from build123d import *

# Parameters (mm, degrees)
SKETCH008_R          = 10.15
SKETCH008_R_2        = 8.35
PAD006_DEPTH         = 55
SKETCH009_R          = 10.15
POCKET002_DEPTH      = 10.15
POCKET002_DEPTH_BACK = 10.15
SKETCH010_R          = 10.15
POCKET003_DEPTH      = 10.15
POCKET003_DEPTH_BACK = 10.15


with BuildPart() as part:
    # Sketch008 → Pad006 (new body)
    with BuildSketch(Plane.XY):
        Circle(SKETCH008_R)
        Circle(SKETCH008_R_2, mode=Mode.SUBTRACT)
    extrude(amount=PAD006_DEPTH)

    # Sketch009 → Pocket002 (cut, two sides)
    with BuildSketch(Plane.XZ) as pocket002_sk:
        Circle(SKETCH009_R)
    extrude(amount=-POCKET002_DEPTH, mode=Mode.SUBTRACT)
    extrude(pocket002_sk.sketch, amount=POCKET002_DEPTH_BACK, mode=Mode.SUBTRACT)

    # Sketch010 → Pocket003 (cut, two sides)
    with BuildSketch(Plane.YZ) as pocket003_sk:
        Circle(SKETCH010_R)
    extrude(amount=-POCKET003_DEPTH, mode=Mode.SUBTRACT)
    extrude(pocket003_sk.sketch, amount=POCKET003_DEPTH_BACK, mode=Mode.SUBTRACT)


solid = part.part
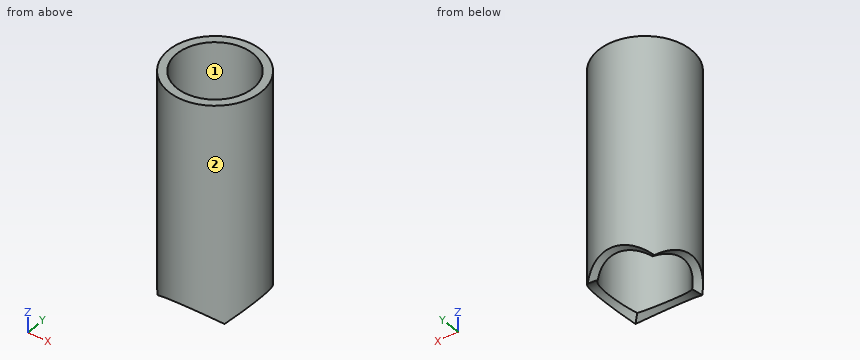
The listing builds one solid part. Answer for the finished solid, in the listing's coordinates (mm). Face numbers are marked on the shaded views. Round coordinates to 2 decimals unless told otherwise and drop trailing zeros. Order: outer loops, then holes, each group sorted by start corner. A loop starts at its lowest first (then second) coordinate and runs counter-clockwise, first axis right, second up. Notation, with made-up numbers: (-10, 12) - (-5, 12) arc R28 cw to (-5, 34) - close; hole circle Ø5 at (16, -29). An arc over 180 degrees is marked (long way). Write item = value, one per line. Start each with the question number.
1) Section B-B, the plane z = 43.5 is taken. Write down the section's boundary in (x, y), plus the area to 3 significant figures.
2) For a pull along X with two mould halves and no side action, classify the marked faces 1 and 2 as released by +X, released by -X, zero draft, split by the parting line, or undercut.
3) Given pin 1 (1 mm diameter, centred on y = -8, z = 29.5, fed in from -X); pin 2 (5 mm diameter, centred on x = -0.5, z = 40.5, fed in from -Y); pin 3 (1.5 mm diameter, centred on y = 3.5, z = 31, fed in from +X); pin 4 (1.5 mm diameter, centred on y = -2.5, z = 47, fed in from +X), each flat-ended and moving along its own axis, determine where each tip first touches the part or whether it passes through.
4) Straight lines are drawn through the part: L1, parallel to Y at x = 0, z = 18; L2, parallel to X at y = 3, z = 21; L3, parallel to X at y = 4.25, z = 13. For each, find the intervals that lie inside material, in ascending order.
5) Section C-C, the plane x = -5.25 is taken. Write down the section's boundary in (y, z).
6) Section A-A, the plane x = 0 is taken. Write down the section's boundary in (y, z), plus the area to 3 significant figures.
Results list:
q1.outline = circle Ø20.3 at (0, 0); hole circle Ø16.7 at (0, 0)
q1.area = 105 mm^2
q2.face_1 = undercut
q2.face_2 = split by the parting line
q3.pin_1 = -6.84
q3.pin_2 = -10.15
q3.pin_3 = 9.77
q3.pin_4 = 10
q4.L1 = -10.15 to -8.35, 8.35 to 10.15
q4.L2 = -9.7 to -7.79, 7.79 to 9.7
q4.L3 = -9.22 to -7.19, 7.19 to 9.22
q5.outline = (-8.69, 8.69) - (-6.49, 8.69) - (-6.49, 55) - (-8.69, 55) - close; (6.49, 8.69) - (8.69, 8.69) - (8.69, 55) - (6.49, 55) - close
q6.outline = (-10.15, 10.15) - (-8.35, 10.15) - (-8.35, 55) - (-10.15, 55) - close; (8.35, 10.15) - (10.15, 10.15) - (10.15, 55) - (8.35, 55) - close
q6.area = 161 mm^2
